Input: part model. Units: mm. Frame: model coordinates. A direction names the side the tool comes from. Round coordinates to 2 decimals unless told otherwise and drop trailing zeros. Order: outer loops, then holes, each group sorted by start corner. A loop starts at its lowest first (then second) coordinate and runs counter-clockwise, first axis right, second up. Notation, with made-up numbers: (87, 34.5) -> (138, 34.5) arc R33 cw to (138, 62.5) -> close; hole circle Ø4 at (38.25, 79.5). An arc over 180 degrees is marked (long way). Use a Markdown table: item, result.
from build123d import *

# Parameters (mm, degrees)
F0_R     = 23.1578344668
F1_DEPTH = 25.4


with BuildPart() as f1:
    # F0 (on Front) → F1 (new body)
    with BuildSketch(Plane.XZ):
        with BuildLine():
            ThreePointArc((-18.6059433036, 47.5486456469), (-28.7840919078, -42.1726319087), (51.059326563, 0))
            ThreePointArc((51.059326563, 0), (42.1726319087, 28.7840919078), (18.6059433036, 47.5486456469))
            Line((18.6059433036, 47.5486456469), (18.6059433036, 40.709229527))
            Line((18.6059433036, 40.709229527), (-18.6059433036, 40.709229527))
            Line((-18.6059433036, 40.709229527), (-18.6059433036, 47.5486456469))
        make_face()
        Circle(F0_R, mode=Mode.SUBTRACT)
        with BuildLine():
            Line((18.6059433036, 40.709229527), (18.6059433036, 47.5486456469))
            ThreePointArc((18.6059433036, 47.5486456469), (0, 51.059326563), (-18.6059433036, 47.5486456469))
            Line((-18.6059433036, 47.5486456469), (-18.6059433036, 40.709229527))
            Line((-18.6059433036, 40.709229527), (18.6059433036, 40.709229527))
        make_face()
        with BuildLine():
            ThreePointArc((-18.6059433036, 47.5486456469), (0, 51.059326563), (18.6059433036, 47.5486456469))
            Line((18.6059433036, 47.5486456469), (18.6059433036, 92.5802945773))
            Line((18.6059433036, 92.5802945773), (-18.6059433036, 92.5802945773))
            Line((-18.6059433036, 92.5802945773), (-18.6059433036, 47.5486456469))
        make_face()
    extrude(amount=F1_DEPTH)


solid = f1.part
1) Cut plane A-A on x = 0. Return loops of the section in (y, z).
Answer key:
| item | result |
|---|---|
| outline | (-25.4, -51.06) -> (0, -51.06) -> (0, -23.16) -> (-25.4, -23.16) -> close; (-25.4, 23.16) -> (0, 23.16) -> (0, 92.58) -> (-25.4, 92.58) -> close |
2) Ray query, probe 1 along Z at (x, y) = (0, -14.75); probe 2 along X at (y, z) = (-20, 19.5); probe 3 along X at (y, z) = (-23, 81.5). Return the intervals inside material, ascending.
Answer key:
| item | result |
|---|---|
| probe 1 | z = -51.06 to -23.16, 23.16 to 92.58 |
| probe 2 | x = -47.19 to -12.49, 12.49 to 47.19 |
| probe 3 | x = -18.61 to 18.61 |
3) Contact query for flat-ended pins moving along their axis: P1, Ø6, axis at x = 38, y = -3, coming from the +Z side; P2, Ø10, axis at y = -14.5, z = -7.5, coming from the +X side; P3, Ø10, axis at y = -7.5, z = 58.5, coming from the -X side. Output: stop coordinate, or through.
Answer key:
| item | result |
|---|---|
| P1 | stops at z = 37.18 |
| P2 | stops at x = 51 |
| P3 | stops at x = -18.61 |
4) Draft query along Z for faces 3 (the face through (0, -13, 92.58)), 4 (the face through (-5.02, -12.522, -22.607)), 5 (the face through (-18.606, -13, 70)). Return one class per face: released by +Z, released by -Z, zero draft, split by the parting line, or undercut.
Answer key:
| item | result |
|---|---|
| face 3 | released by +Z |
| face 4 | undercut |
| face 5 | zero draft |
5) Cut plane D-D on z = -26. Return loops of the section in (x, y).
Answer key:
| item | result |
|---|---|
| outline | (-43.94, -25.4) -> (43.94, -25.4) -> (43.94, 0) -> (-43.94, 0) -> close |
6) Set-up query: faces 1 (the face through (18.606, -13, 70)), 2 (the face through (11, 0, 22)). Return all of +Z, -Z, +X, -X, +Y, -Y with unobstructed straight access to the full face (end or side cutting, diameter ignored); none if empty.
Answer key:
| item | result |
|---|---|
| face 1 | +Z, +X, +Y, -Y |
| face 2 | +Z, -Z, +X, -X, +Y |
7) Cut plane C-C on z = -9. Return loops of the section in (x, y).
Answer key:
| item | result |
|---|---|
| outline | (-50.26, -25.4) -> (-21.34, -25.4) -> (-21.34, 0) -> (-50.26, 0) -> close; (21.34, -25.4) -> (50.26, -25.4) -> (50.26, 0) -> (21.34, 0) -> close |
8) Cut plane B-B on y = -18.75. Return loops of the section in (x, z).
Answer key:
| item | result |
|---|---|
| outline | (-18.61, 47.55) arc R51.06 ccw (long way) to (18.61, 47.55) -> (18.61, 92.58) -> (-18.61, 92.58) -> close; hole circle Ø46.32 at (0, 0) |
